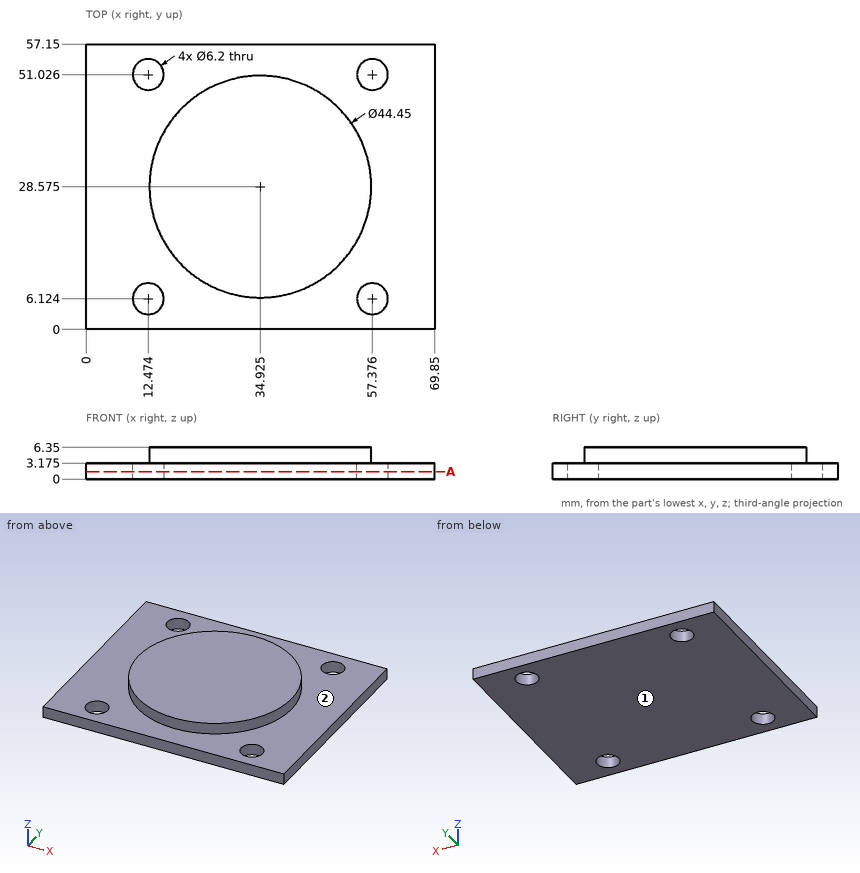
Here's the drawing with two shaded views (mm, measured from the low corner). I have some questions. A direction names the side the tool comes from. Round coordinates to 2 decimals unless told otherwise and drop trailing zeros. Write each question's results on one line, items separated by ' | '. Start each with the question number.
1. I'm going to push flat-ended pins straight in: pin 1 Ø1.5 at (x, z) = (14.5, 4.5) entering from +Y; pin 2 Ø8 at (x, y) = (12.47, 51.03) entering from +Z (3 decimals); pin 3 Ø10 at (x, y) = (57.38, 51.03) entering from -Z. Where does each tip first touch, or does it pass through?
2. Imagine slicing it at A-A on z = 1.5. Count the separate pieces of the cut face and the enclosed holes in it, and give its area (3 significant figures).
3. On a 3-axis mill with a long thin cutter (end or side, diameter ignored), from which of +Z, -Z, +X, -X, +Y, -Y can I reach the whole of each face in a straight line? I mean the marked faces 1 and 2. Say none if no direction works.
4. I need wall thicknesses on L1, parallel to Z at x = 10, y = 42 (1 decimal); L2, parallel to Y at x = 24, z = 6; L3, parallel to X at y = 51.5, z = 2.75. Which ranges of each line are inside material? Lowest first, please. Write a range as from..to.
Result sheet:
1) pin 1: stops at y = 38.91 | pin 2: stops at z = 3.175 | pin 3: stops at z = 0
2) separate pieces: 1 | enclosed holes: 4 | area: 3,870 mm^2
3) face 1: -Z, +X, -X, +Y, -Y | face 2: +Z
4) L1: z = 0..3.2 | L2: y = 9.22..47.93 | L3: x = 0..9.41, 15.54..54.31, 60.44..69.85
